For this review, take the finished solid that the model builds, in its own axes (mm). A direction names the side the tool comes from. Coordinates: 2 decimals unless noted, no trailing zeros. Write each loop counter-clockwise with the first axis right and the second up, starting at its lowest first coordinate (ties: lowest second). Pieces come first, ordered by that corner, then holes. Notation, with made-up numbers: M 51.5,44.5 L 98.5,44.5 A32 cw 98.5,78.5 Z; hole C 53,71 d4. An arc over 180 degrees is marked long. One line per question, with ' | ' between items.
from build123d import *

# Parameters (mm, degrees)
CROQUIS1_R              = 20
CROQUIS1_R_2            = 12.789172095
SALIENTE_EXTRUIR1_DEPTH = 2.5
CROQUIS2_R              = 15.5
CROQUIS2_R_2            = 12.789172095
SALIENTE_EXTRUIR2_DEPTH = 15
CORTAR_EXTRUIR1_START   = -14
CORTAR_EXTRUIR1_DEPTH   = 14
MATRIZC1_COUNT          = 3
CROQUIS4_R              = 2
CORTAR_EXTRUIR2_DEPTH   = 17


with BuildPart() as part:
    # Croquis1 → Saliente-Extruir1 (new body)
    with BuildSketch(Plane(origin=(0, 0, 0), x_dir=(1, 0, 0), z_dir=(0, 1, 0))):
        with Locations(Location((0, 0, 0), (0, 0, 270))):
            Circle(CROQUIS1_R)
        with Locations(Location((0, 0, 0), (0, 0, 270))):
            Circle(CROQUIS1_R_2, mode=Mode.SUBTRACT)
    extrude(amount=SALIENTE_EXTRUIR1_DEPTH)

    # Croquis2 → Saliente-Extruir2 (add)
    with BuildSketch(Plane(origin=(0, 2.5, 0), x_dir=(1, 0, 0), z_dir=(0, 1, 0))):
        with Locations(Location((0, 0, 0), (0, 0, 270))):
            Circle(CROQUIS2_R)
        with Locations(Location((0, 0, 0), (0, 0, 270))):
            Circle(CROQUIS2_R_2, mode=Mode.SUBTRACT)
    extrude(amount=SALIENTE_EXTRUIR2_DEPTH)

    # Croquis3 → Cortar-Extruir1 (cut)
    with BuildSketch(Plane(origin=(0, 17.5, 0), x_dir=(1, 0, 0), z_dir=(0, 1, 0)).offset(CORTAR_EXTRUIR1_START)):
        with BuildLine():
            Line((2, 15.370426149), (2, 12.631821835))
            ThreePointArc((2, 12.631821835), (0, 12.789172095), (-2, 12.631821835))
            Line((-2, 12.631821835), (-2, 15.370426149))
            ThreePointArc((-2, 15.370426149), (0, 15.5), (2, 15.370426149))
        make_face()
    cortar_extruir1 = extrude(amount=CORTAR_EXTRUIR1_DEPTH, mode=Mode.SUBTRACT)

    # MatrizC1: Cortar-Extruir1 ×3 about axis
    matrizc1_axis = Axis((0, 0, 0), (0, 1, 0))
    for i in range(1, MATRIZC1_COUNT):
        add(cortar_extruir1.rotate(matrizc1_axis, i * 360 / MATRIZC1_COUNT), mode=Mode.SUBTRACT)

    # Croquis4 → Cortar-Extruir2 (cut)
    with BuildSketch(Plane(origin=(0, 0, 0), x_dir=(0.7071067811865477, 0, 0.7071067811865475), z_dir=(-0.7071067811865475, 0, 0.7071067811865477))):
        with Locations((0, 6.5)):
            Circle(CROQUIS4_R)
    extrude(amount=-CORTAR_EXTRUIR2_DEPTH, mode=Mode.SUBTRACT)


solid = part.part
1) We need section B-B on y = 15.25. State the section outline as (x, z) points, then the cut area to 3 significant figures.
Responses:
outline: M -14.31,5.95 A15.5 ccw -2,-15.37 L -2,-12.63 A12.79 cw -11.94,4.58 Z; M -12.31,9.42 L -9.94,8.05 A12.79 cw 9.94,8.05 L 12.31,9.42 A15.5 ccw Z; M 2,-15.37 A15.5 ccw 14.31,5.95 L 11.94,4.58 A12.79 cw 2,-12.63 Z | area: 208 mm^2
2) The part is to be moulded in two halves that separate along Z. For faces 1 (the cylindrical face through (-5.937, 9.895, 14.318)), 2 (the flat face through (-11, 17.5, -7)), 3 (the flat face through (11.14, 10.4, 8.74)), say which applies: +Z half, -Z half, draft (parallel to the pull), parting line (faces both ways), or undercut.
Responses:
face 1: parting line | face 2: draft | face 3: undercut
3) Insertion check: pin 1 Ø4 at (x, y) = (1, 7) entering from +Z; pin 2 Ø3 at (y, z) = (12.5, -13.5) entering from -X; pin 3 Ø3.5 at (x, z) = (12.5, 7) entering from +Y. Each pin has a flat end and moves straight along its axis. Give the tip position at first contact, or say it passes through.
Responses:
pin 1: z = 15.5 | pin 2: x = -9.81 | pin 3: y = 3.5
4) We need section C-C on x = 0. State the section outline as (y, z) points, then the cut area to 3 significant figures.
Responses:
outline: M 0,-20 L 2.5,-20 L 2.5,-15.5 L 3.5,-15.5 L 3.5,-12.79 L 0,-12.79 Z; M 0,12.79 L 17.5,12.79 L 17.5,15.5 L 2.5,15.5 L 2.5,20 L 0,20 Z | area: 79.4 mm^2
5) We need section D-D on y = 6. State the section outline as (x, z) points, then the cut area to 3 significant figures.
Responses:
outline: M -14.31,5.95 A15.5 ccw -2,-15.37 L -2,-12.63 A12.79 cw -11.94,4.58 Z; M -12.31,9.42 L -9.94,8.05 A12.79 cw 9.94,8.05 L 12.31,9.42 A15.5 ccw Z; M 2,-15.37 A15.5 ccw 9.5,-12.24 L 7.57,-10.31 A12.79 cw 2,-12.63 Z; M 10.31,-7.57 L 12.24,-9.5 A15.5 ccw 14.31,5.95 L 11.94,4.58 A12.79 cw Z | area: 198 mm^2
6) Machinability: for faces 4 (the flat face through (0, 3.5, -14)), 5 (the flat face through (-11.8, 2.5, 10.3)), 6 (the flat face through (-11.109, 10.402, 8.723)), 7 (the cylindrical face through (-4.898, 8.628, 11.814)), which of the approach directions +Z, -Z, +X, -X, +Y, -Y give a long, thin tool a straight path to every point of the face, cutting with its end or side? Answer none if there is none.
Responses:
face 4: -Z, +Y | face 5: +Y | face 6: -X, +Y | face 7: +Y, -Y
7) We need section A-A on z = 0. State the section outline as (x, y) points, then the cut area to 3 significant figures.
Responses:
outline: M -20,0 L -12.79,0 L -12.79,17.5 L -15.5,17.5 L -15.5,2.5 L -20,2.5 Z; M 12.79,0 L 20,0 L 20,2.5 L 15.5,2.5 L 15.5,17.5 L 12.79,17.5 Z | area: 117 mm^2
8) To check wall thickness, follow line 1 along X through (y, z) = (10.5, 0); line 2 along Y through (x, z) = (16, -6); line 3 along Z through (x, y) = (0, 4.25). State the ranges of each line that lie inside material, in increasing order. Write a range as [from, to].
Responses:
line 1: [-15.5, -12.79], [12.79, 15.5] | line 2: [0, 2.5] | line 3: [12.79, 15.5]
